from build123d import *

# Parameters (mm, degrees)
EXTRUDE_1_DEPTH = 4
SKETCH_2_R      = 4
EXTRUDE_2_DEPTH = 20


with BuildPart() as part:
    # 草图1 → 凸台-拉伸1 (new body)
    with BuildSketch(Plane(origin=(0, 0, 0), x_dir=(1, 0, 0), z_dir=(0, 1, 0))):
        Polygon((3.419107318, 6.025753492), (-3.508901942, 5.973910542), (-6.92800926, -0.05184295), (-3.419107318, -6.025753492), (3.508901942, -5.973910542), (6.92800926, 0.05184295), align=None)
    extrude(amount=EXTRUDE_1_DEPTH)

    # 草图2 → 凸台-拉伸2 (add)
    with BuildSketch(Plane(origin=(0, 4, 0), x_dir=(1, 0, 0), z_dir=(0, 1, 0))):
        with Locations(Location((0, 0, 0), (0, 0, 270))):
            Circle(SKETCH_2_R)
    extrude(amount=EXTRUDE_2_DEPTH)

    # 草图5 → 切除-旋转3 (revolve, cut)
    with BuildSketch(Plane(origin=(0, 0, 0), x_dir=(0.4935056326713254, 0, -0.8697426001534447), z_dir=(0.8697426001534447, 0, 0.4935056326713254)), mode=Mode.PRIVATE) as cut_revolve_3_sk:
        Polygon((6.92820323, 0.5), (5.72820323, 0), (6.92820323, 0), align=None)
    revolve(cut_revolve_3_sk.sketch.rotate(Axis((0, -1000, 0), (0, 1, 0)), 179.999999998), axis=Axis((0, -1000, 0), (0, 1, 0)), mode=Mode.SUBTRACT)


solid = part.part
Input: part model. Units: mm. Frame: model coordinates. A direction names the side the tool comes from. Coordinates: 2 decimals unless noted, no trailing zeros. Write each loop counter-clockwise with the first axis right and the second up, starting at its lowest first coordinate (ties: lowest second). Pieces come first, ordered by that corner, then holes. Notation, with made-up numbers: M -23,26.25 L 27,26.25 A15 cw 27,39.25 Z; hole C -10.5,52.25 d11. An arc over 180 degrees is marked long. Answer as a JSON object with one key per item and string values. Group by question number.
(1) Section B-B on x = 0. Output: boundary loops of the cut face in (y, z).
(2) Section A-A on y = 2. Output: boundary loops of the cut face in (x, z), plus the area to 3 significant figures.
(3) Set-up query: faces 1 (the face through (0, 24, 0)), 2 (the face through (-3.905, 13.86, -0.867)). Return all of +Z, -Z, +X, -X, +Y, -Y with unobstructed straight access to the full face (end or side cutting, diameter ignored); none if empty.
(4) Contact query for flat-ended pins moving along their axis: P1, Ø1, axis at x = -0.5, z = 0.5, coming from the -Y side; P2, Ø6, axis at y = 8, z = 1.5, coming from the -X side; P3, Ø3, axis at y = 19, z = -1, coming from the +X side; P4, Ø3, axis at x = -4, y = 4, coming from the -Z side. Output: stop coordinate, or through.
(5) Ray query, line 1 along X through (y, z) = (5.25, 0); line 2 along Y through (x, z) = (-4, -1); line 3 along Z through (x, y) = (3.5, 9.5). Return the intervals inside material, ascending. Write a range as [from, to].
(6) Section C-C on y = 18.75. Output: boundary loops of the cut face in (x, z), plus the area to 3 significant figures.
Result set:
{
 "1": {"outline": "M 0,-5.73 L 0.11,-6 L 4,-6 L 4,-4 L 24,-4 L 24,4 L 4,4 L 4,6 L 0.11,6 L 0,5.73 Z"},
 "2": {"outline": "M -6.93,0.05 L -3.51,-5.97 L 3.42,-6.03 L 6.93,-0.05 L 3.51,5.97 L -3.42,6.03 Z", "area": "125 mm2"},
 "3": {"face 1": "+Z, -Z, +X, -X, +Y", "face 2": "+Y"},
 "4": {"P1": "stops at y = 0", "P2": "stops at x = -4", "P3": "stops at x = 4", "P4": "stops at z = -5.98"},
 "5": {"line 1": "x = [-4, 4]", "line 2": "y = [0, 4]", "line 3": "z = [-1.94, 1.94]"},
 "6": {"outline": "C 0,0 d8", "area": "50.3 mm2"}
}
